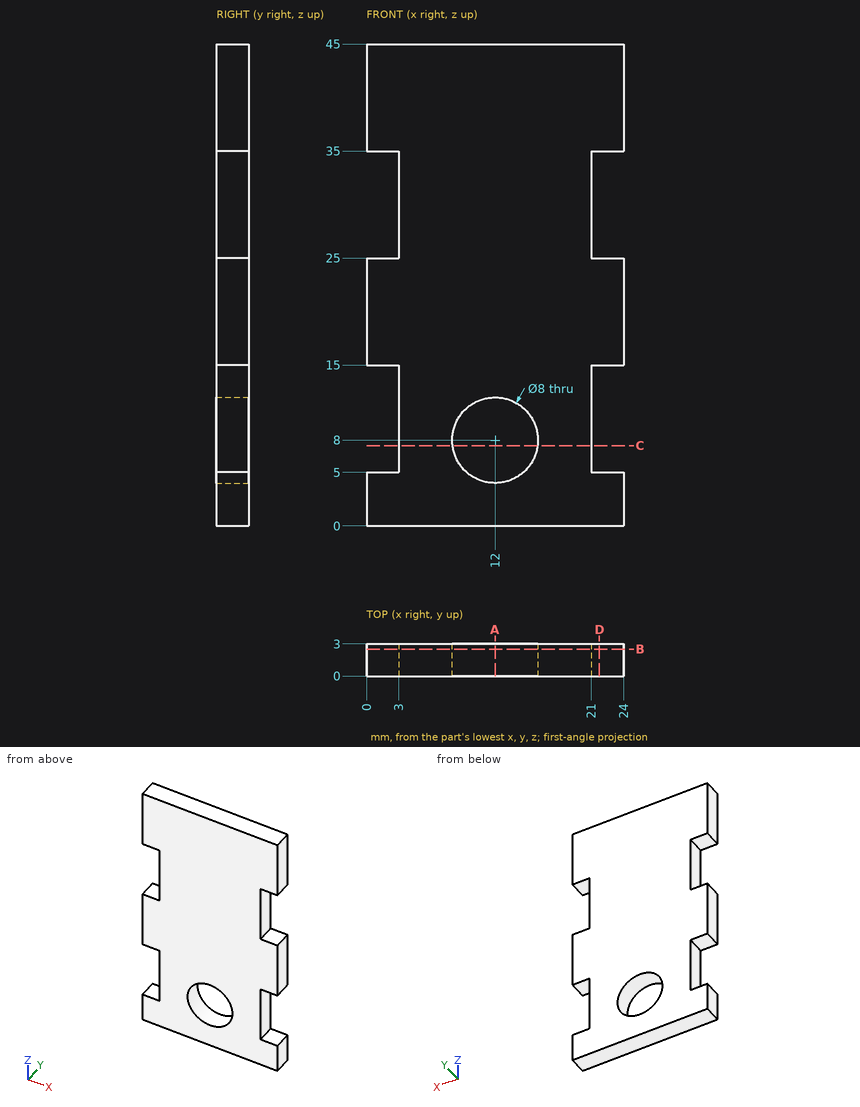
Part print with two shaded views. Sizes in mm from the minimum x, y, z corner. Round coordinates to 2 decimals unless told otherwise and drop trailing zeros. Order: outer loops, then holes, each group sorted by start corner. A loop starts at its lowest first (then second) coordinate and runs counter-clockwise, first axis right, second up. Notation, with made-up numbers: M 52.25,1.5 L 61.25,1.5 A20 cw 61.25,8.5 Z; hole C 20,-26 d9. An arc over 180 degrees is marked long. Put each result on its own line as item: value. Start each with the question number.
1. Slice it at D-D on x = 21.75. List the corners of the cut face in (y, z).
2. Slice it at B-B on y = 2.5. List the corners of the cut face in (x, z).
3. Drill centre lines: probe 1 along Z at (x, y) = (21.5, 2.55); probe 2 along Z at (x, y) = (12, 2.15); probe 3 along X at (y, z) = (1.5, 8). Where is each one in solid material? Low to high. Write a range as [from, to].
4. Slice it at A-A on x = 12. List the corners of the cut face in (y, z).
5. Drop flat-ended pins along their axis: pin 1 (3 mm diameter, centred on x = 15.5, z = 32.5, fed in from -Y); pin 2 (0.9 mm diameter, centred on y = 2, z = 10.5, fed in from +X); pin 3 (1.5 mm diameter, centred on y = 1, z = 28, fed in from -X). Give the stop position or say it passes through.
6. Slice it at C-C on z = 7.5. List the corners of the cut face in (x, y), then the cut area to 3 significant figures.
Findings:
1. outline: M 0,0 L 3,0 L 3,5 L 0,5 Z; M 0,15 L 3,15 L 3,25 L 0,25 Z; M 0,35 L 3,35 L 3,45 L 0,45 Z
2. outline: M 0,0 L 24,0 L 24,5 L 21,5 L 21,15 L 24,15 L 24,25 L 21,25 L 21,35 L 24,35 L 24,45 L 0,45 L 0,35 L 3,35 L 3,25 L 0,25 L 0,15 L 3,15 L 3,5 L 0,5 Z; hole C 12,8 d8
3. probe 1: [0, 5], [15, 25], [35, 45]
3. probe 2: [0, 4], [12, 45]
3. probe 3: [3, 8], [16, 21]
4. outline: M 0,0 L 3,0 L 3,4 L 0,4 Z; M 0,12 L 3,12 L 3,45 L 0,45 Z
5. pin 1: y = 0
5. pin 2: x = 21
5. pin 3: x = 3
6. outline: M 3,0 L 8.03,0 L 8.03,3 L 3,3 Z; M 15.97,0 L 21,0 L 21,3 L 15.97,3 Z
6. area: 30.2 mm2
